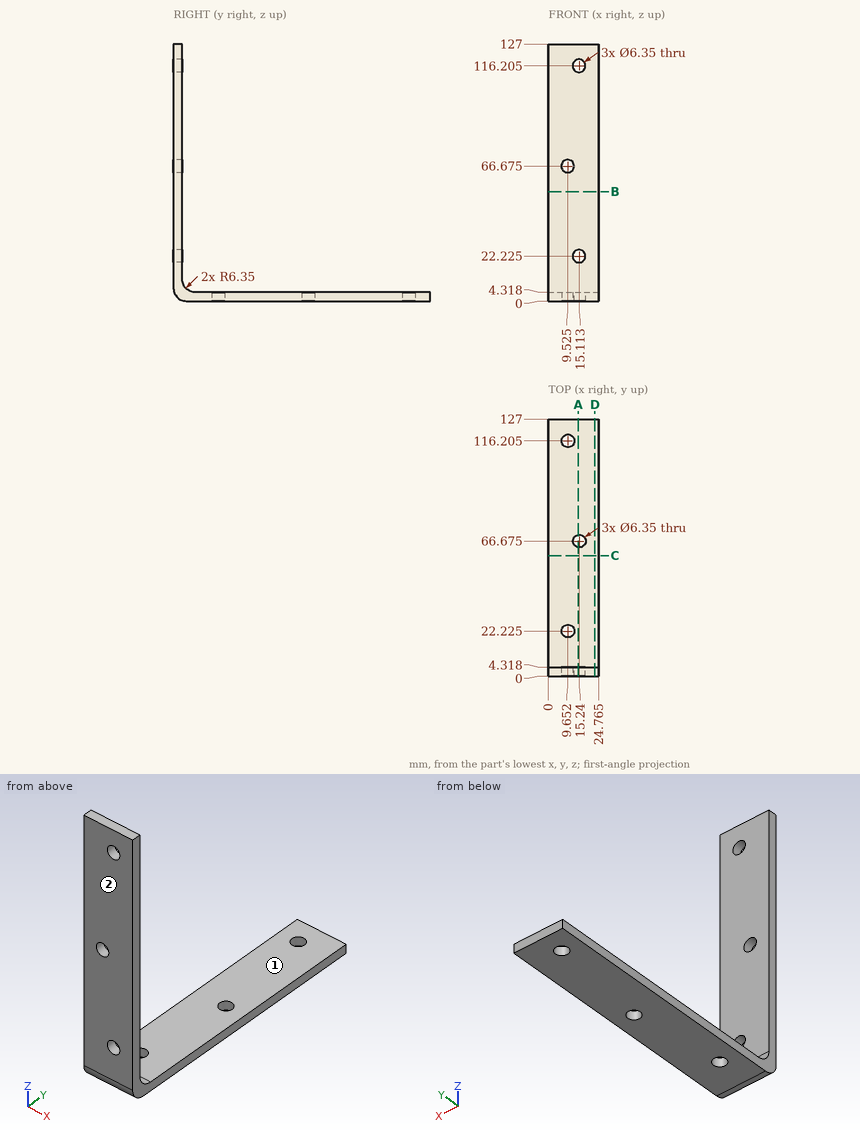
Design review of the part shown in the three views and the two pictorial views. Dimensions are in mm from the part's minimum x, y and z. A direction names the side the tool comes from. Coordinates: 2 decimals unless noted, no trailing zeros. Loops run counter-clockwise (first coordinate to the right, second up) from the corner with the lowest first, then second, coordinate; pieces in that order, holes last.
(1) Consider section D-D, the plane x = 23. Give the boundary of the cut face in (y, z), plus the area to 3 significant figures.
Determined:
outline: (0, 6.35) arc R6.35 ccw to (6.35, 0) - (127, 0) - (127, 4.32) - (10.67, 4.32) arc R6.35 cw to (4.32, 10.67) - (4.32, 127) - (0, 127) - close
area: 1,080 mm2
(2) Insertion check: P1, Ø7.5, axis at x = 12, z = 72.5, coming from the +Y side; P2, Ø7.5, axis at x = 9.652, y = 22.225, coming from the -Z side; P3, Ø5, axis at x = 9.525, z = 66.675, coming from the -Y side; P4, Ø1.5, axis at x = 3.5, y = 102.5, coming from the +Z side. Each pin has a flat end and moves straight along its axis. Give the tip position at first contact, or say it passes through.
Determined:
P1: stops at y = 4.32
P2: stops at z = 0
P3: passes through
P4: stops at z = 4.32
(3) Consider section B-B, the plane z = 54. Give the boundary of the cut face in (x, y) (3 decimals), plus the area to 3 significant figures.
Determined:
outline: (0, 0) - (24.765, 0) - (24.765, 4.318) - (0, 4.318) - close
area: 107 mm2
(4) Consider section A-A, the plane x = 14.75. Give the boundary of the cut face in (y, z), plus the area to 3 significant figures.
Determined:
outline: (0, 6.35) arc R6.35 ccw to (6.35, 0) - (63.54, 0) - (63.54, 4.32) - (10.67, 4.32) arc R6.35 cw to (4.32, 10.67) - (4.32, 19.07) - (0, 19.07) - close; (0, 25.38) - (4.32, 25.38) - (4.32, 113.05) - (0, 113.05) - close; (0, 119.36) - (4.32, 119.36) - (4.32, 127) - (0, 127) - close; (69.81, 0) - (127, 0) - (127, 4.32) - (69.81, 4.32) - close
area: 997 mm2
(5) Tool access review of the marked faces 1 and 2: name each direction out of +Z, -Z, +X, -X, +Y, -Y from which nothing blocks a thin tool from reaching the whole face with its end or side.
Determined:
face 1: +Z, +X, -X, +Y
face 2: +Z, -Z, +X, -X, -Y
(6) Wall thickness on L1, parallel to Y at x = 2.5, z = 28; L2, parallel to Y at x = 15.24, z = 2.4: over which ranges is each line inside the solid? List them lowest first.
Determined:
L1: y = 0 to 4.32
L2: y = 1.38 to 63.5, 69.85 to 127
